Print and shaded views of the part. All mm, measured from the part's lowest x, y and z. Round coordinates to 2 decimals unless told otherwise and drop trailing zeros. Loops run counter-clockwise (first coordinate to the right, second up) from the corner with the lowest first, then second, coordinate; pieces in that order, holes last. Notation, with made-up numbers: (-7, 11.5) - (33, 11.5) arc R25 ccw to (33, 41.5) - close; hole circle Ø11 at (-18.75, 40.25). An arc over 180 degrees is marked (long way). Answer as a JSON object with one key per item and string values.
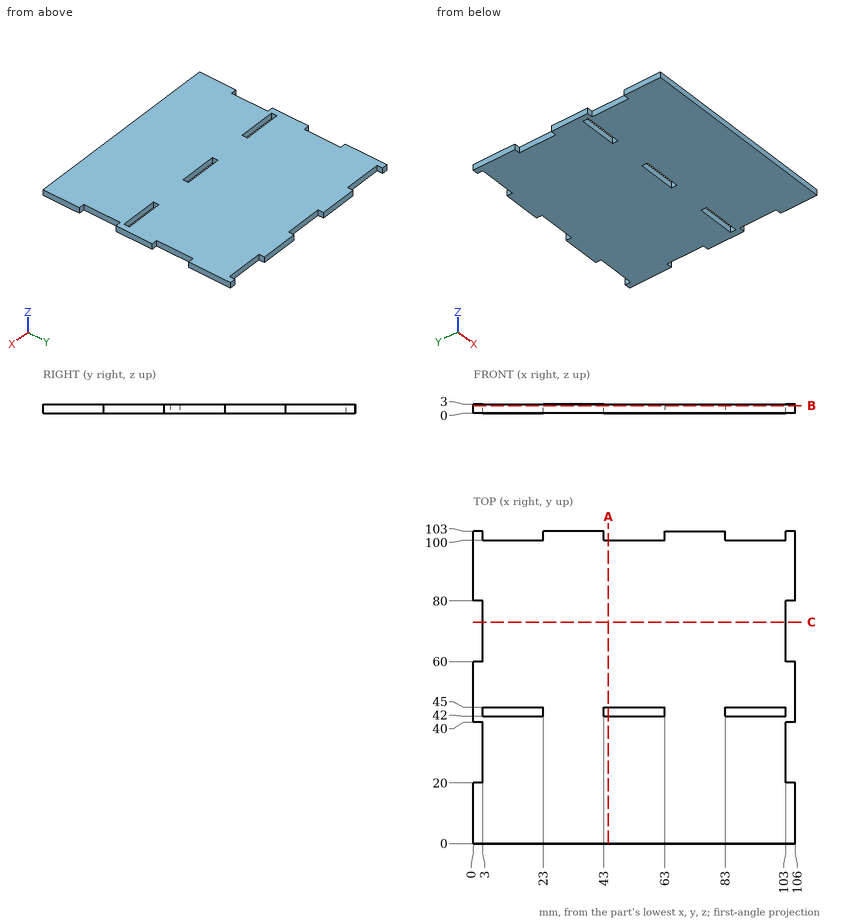
1) Drop a flat-ended pin along its axis: P1, Ø0.9, axis at x = 9, z = 2, coming from the +Y side. Give the stop position or say it passes through.
Values follow:
{"P1": "y = 100"}
2) Probe probe 1 along Y at (x, z) = (55.5, 1.7); probe 2 along X at (y, z) = (71, 2.1). List the from-to ranges inside material, lowest first.
Values follow:
{"probe 1": "0 to 42, 45 to 100", "probe 2": "3 to 103"}
3) Slice it at A-A on x = 44.5. List the corners of the cut face in (y, z).
Values follow:
{"outline": "(0, 0) - (42, 0) - (42, 3) - (0, 3) - close; (45, 0) - (100, 0) - (100, 3) - (45, 3) - close"}
4) Slice it at C-C on y = 73. List the corners of the cut face in (x, z).
Values follow:
{"outline": "(3, 0) - (103, 0) - (103, 3) - (3, 3) - close"}
5) Slice it at B-B on z = 2.5. Count the separate pieces of the cut face and the enclosed holes in it, then the cut area to 3 significant figures.
Values follow:
{"separate pieces": "1", "enclosed holes": "3", "area": "10,300 mm²"}
